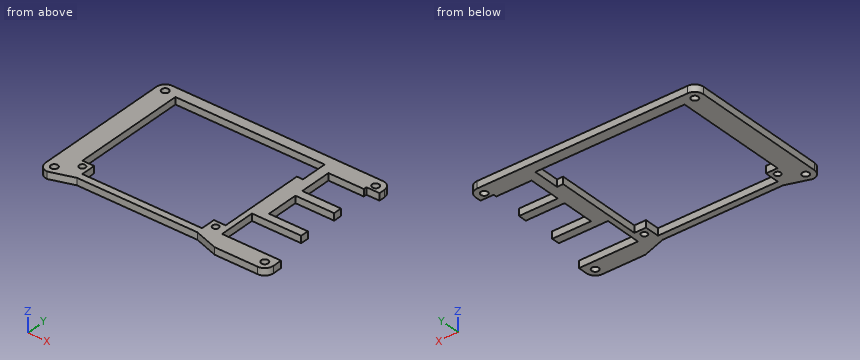
```python
from build123d import *

# Parameters (mm, degrees)
SKETCH1_R           = 1.524
SKETCH1_W           = 60.6932
SKETCH1_H           = 7.81
SKETCH1_W_2         = 5.588
SKETCH1_H_2         = 23.368
SKETCH1_W_3         = 5.4034
SKETCH1_H_3         = 22.6066
BOSS_EXTRUDE1_DEPTH = 3.048
SKETCH2_R           = 10.922
SKETCH2_R_2         = 1.4986
CUT_EXTRUDE1_DEPTH  = 4.048
SKETCH3_W           = 60.6932
SKETCH3_H           = 56.8638
BOSS_EXTRUDE2_DEPTH = 3.048
SKETCH5_W           = 64.8849
SKETCH5_H           = 11.62
SKETCH5_R           = 2.7305
CUT_EXTRUDE3_DEPTH  = 4.048
SKETCH6_R           = 2.7305
SKETCH6_R_2         = 1.35255
BOSS_EXTRUDE3_DEPTH = 3.048
SKETCH7_W           = 15.3651
SKETCH7_H           = 1.397
BOSS_EXTRUDE4_DEPTH = 3.048
SKETCH8_W           = 52.07
SKETCH8_H           = 6.35
CUT_EXTRUDE4_DEPTH  = 4.048


with BuildPart() as part:
    # Sketch1 → Boss-Extrude1 (new body)
    with BuildSketch(Plane.XY):
        with BuildLine():
            Line((61.214907375, 24.068294304), (40.134807375, 24.068294304))
            Line((40.134807375, 24.068294304), (40.134807375, 8.658194304))
            Line((40.134807375, 8.658194304), (56.975007375, 8.658194304))
            Line((56.975007375, 8.658194304), (56.975007375, 4.997894304))
            Line((56.975007375, 4.997894304), (40.134807375, 4.997894304))
            Line((40.134807375, 4.997894304), (40.134807375, -9.121805696))
            Line((40.134807375, -9.121805696), (56.975007375, -9.121805696))
            Line((56.975007375, -9.121805696), (56.975007375, -12.628005696))
            Line((56.975007375, -12.628005696), (35.575007375, -12.628005696))
            Line((35.575007375, -12.628005696), (35.575007375, -28.627805696))
            Line((35.575007375, -28.627805696), (61.214907375, -28.627805696))
            Line((61.214907375, -28.627805696), (61.214907375, -32.613401529))
            ThreePointArc((61.214907375, -32.613401529), (60.108826144, -35.325305244), (57.405007375, -36.451005696))
            Line((57.405007375, -36.451005696), (38.714307375, -36.451005696))
            Line((38.714307375, -36.451005696), (28.474307375, -33.084405696))
            Line((28.474307375, -33.084405696), (-23.844892625, -33.084405696))
            Line((-23.844892625, -33.084405696), (-34.084892625, -36.451005696))
            ThreePointArc((-34.084892625, -36.451005696), (-36.778969461, -35.335082532), (-37.894892625, -32.641005696))
            Line((-37.894892625, -32.641005696), (-37.894892625, 26.697694304))
            ThreePointArc((-37.894892625, 26.697694304), (-36.778969461, 29.391771141), (-34.084892625, 30.507694304))
            Line((-34.084892625, 30.507694304), (57.404932375, 30.507694304))
            ThreePointArc((57.404932375, 30.507694304), (60.103884597, 29.386886916), (61.214907375, 26.683892153))
            Line((61.214907375, 26.683892153), (61.214907375, 24.068294304))
        make_face()
        with Locations((57.405007375, -32.641005696)):
            Circle(SKETCH1_R, mode=Mode.SUBTRACT)
        with Locations((-34.084892625, -32.641005696)):
            Circle(SKETCH1_R, mode=Mode.SUBTRACT)
        with Locations((-34.084892625, 26.697694304)):
            Circle(SKETCH1_R, mode=Mode.SUBTRACT)
        with Locations((57.404932375, 26.697694304)):
            Circle(SKETCH1_R, mode=Mode.SUBTRACT)
        with Locations((1.341707375, 21.991994304)):
            Rectangle(SKETCH1_W, SKETCH1_H, mode=Mode.SUBTRACT)
        with Locations((-26.210892625, -1.882805696)):
            Rectangle(SKETCH1_W_2, SKETCH1_H_2, mode=Mode.SUBTRACT)
        with Locations((16.546707375, -19.663505696)):
            Rectangle(SKETCH1_W_3, SKETCH1_H_3, mode=Mode.SUBTRACT)
    extrude(amount=BOSS_EXTRUDE1_DEPTH)

    # Sketch2 → Cut-Extrude1 (cut, through all)
    with BuildSketch(Plane.XY.offset(3.048)):
        with Locations((-0.302892625, -0.480305696)):
            Circle(SKETCH2_R)
        with Locations((-10.285092625, -10.462505696)):
            Circle(SKETCH2_R_2)
        with Locations((-10.285092625, 9.501894304)):
            Circle(SKETCH2_R_2)
        with Locations((9.679307375, -10.462505696)):
            Circle(SKETCH2_R_2)
        with Locations((9.679307375, 9.501894304)):
            Circle(SKETCH2_R_2)
    extrude(amount=-CUT_EXTRUDE1_DEPTH, mode=Mode.SUBTRACT)

    # Sketch3 → Boss-Extrude2 (add)
    with BuildSketch(Plane.XY.offset(3.048)):
        with Locations((1.341707375, -2.534905696)):
            Rectangle(SKETCH3_W, SKETCH3_H)
    extrude(amount=-BOSS_EXTRUDE2_DEPTH)

    # Sketch5 → Cut-Extrude3 (cut, through all)
    with BuildSketch(Plane.XY.offset(3.048)):
        with Locations((3.437557375, 20.086994304)):
            Rectangle(SKETCH5_W, SKETCH5_H)
        with Locations((-26.839542625, -26.572455696)):
            Circle(SKETCH5_R)
        with Locations((31.135957375, -26.572455696)):
            Circle(SKETCH5_R)
    extrude(amount=-CUT_EXTRUDE3_DEPTH, mode=Mode.SUBTRACT)

    # Sketch6 → Boss-Extrude3 (add)
    with BuildSketch(Plane.XY.offset(3.048)):
        with Locations((-26.839542625, -26.572455696)):
            Circle(SKETCH6_R)
        with Locations((-26.839542625, -26.572455696)):
            Circle(SKETCH6_R_2, mode=Mode.SUBTRACT)
        with Locations((31.135957375, -26.572455696)):
            Circle(SKETCH6_R)
        with Locations((31.135957375, -26.572455696)):
            Circle(SKETCH6_R_2, mode=Mode.SUBTRACT)
    extrude(amount=-BOSS_EXTRUDE3_DEPTH)

    # Sketch7 → Boss-Extrude4 (add)
    with BuildSketch(Plane.XY.offset(3.048)):
        with Locations((47.817357375, 23.369794304)):
            Rectangle(SKETCH7_W, SKETCH7_H)
    extrude(amount=-BOSS_EXTRUDE4_DEPTH)

    # Sketch8 → Cut-Extrude4 (cut, through all)
    with BuildSketch(Plane.XY.offset(3.048)):
        Polygon((-29.004892625, -23.823005696), (-23.924892625, -23.823005696), (28.145107375, -23.823005696), (33.225107375, -23.823005696), (33.225107375, 14.276994304), (-29.004892625, 14.276994304), align=None)
        with Locations((2.110107375, -26.998005696)):
            Rectangle(SKETCH8_W, SKETCH8_H)
    extrude(amount=-CUT_EXTRUDE4_DEPTH, mode=Mode.SUBTRACT)


solid = part.part
```
Part model, mm, in its own coordinate system. Coordinates: 2 decimals unless noted, no trailing zeros. Order: outer loops, then holes, each group sorted by start corner. A loop starts at its lowest first (then second) coordinate and runs counter-clockwise, first axis right, second up. Notation, with made-up numbers: (86.25, 7) - (111.25, 7) arc R15 cw to (111.25, 14) - close; hole circle Ø11 at (29.25, 50). An arc over 180 degrees is marked (long way). Return JSON: item names as keys, results as strings. Group by question number.
Item 1: Cut at C-C (x = 6). List the corners of the cut face in (y, z).
Item 2: Cut at A-A (x = 51.5). List the corners of the cut face in (y, z), plus the area to 3 significant figures.
Item 3: Drill centre lines: probe 1 along X at (y, z) = (11, 1.4); probe 2 along X at (y, z) = (-22.5, 2.2) (3 decimals); probe 3 along Y at (x, z) = (6, 2.55). Where is each one in solid material? Low to high. Write a range as from..to.
Item 4: Pin check, flat tip, straight feed: pin 1 (1.5 mm diameter, centred on y = 15, z = 1, fed in from +X). Stop position of the tip, or through.
Item 5: Cut at B-B (y = -15). List the corners of the cut face in (x, z) (3 decimals), plus the area to 3 significant figures.
Item 6: Cut at D-D (x = -26.5). List the corners of the cut face in (y, z), plus the area to 3 significant figures.
Check values:
{
 "1": {"outline": "(-33.08, 0) - (-30.17, 0) - (-30.17, 3.05) - (-33.08, 3.05) - close; (25.9, 0) - (30.51, 0) - (30.51, 3.05) - (25.9, 3.05) - close"},
 "2": {"outline": "(-36.45, 0) - (-28.63, 0) - (-28.63, 3.05) - (-36.45, 3.05) - close; (-12.63, 0) - (-9.12, 0) - (-9.12, 3.05) - (-12.63, 3.05) - close; (5, 0) - (8.66, 0) - (8.66, 3.05) - (5, 3.05) - close; (22.67, 0) - (30.51, 0) - (30.51, 3.05) - (22.67, 3.05) - close", "area": "69.6 mm2"},
 "3": {"probe 1": "x = -37.89..-29, 33.23..40.13", "probe 2": "x = -37.895..-29.005, 33.225..35.575", "probe 3": "y = -33.08..-30.17, 25.9..30.51"},
 "4": {"pin 1": "stops at x = 40.13"},
 "5": {"outline": "(-37.895, 0) - (-29.005, 0) - (-29.005, 3.048) - (-37.895, 3.048) - close; (33.225, 0) - (35.575, 0) - (35.575, 3.048) - (33.225, 3.048) - close", "area": "34.3 mm2"},
 "6": {"outline": "(-33.96, 0) - (-27.88, 0) - (-27.88, 3.05) - (-33.96, 3.05) - close; (-25.26, 0) - (-23.82, 0) - (-23.82, 3.05) - (-25.26, 3.05) - close; (25.9, 0) - (30.51, 0) - (30.51, 3.05) - (25.9, 3.05) - close", "area": "37.0 mm2"}
}
